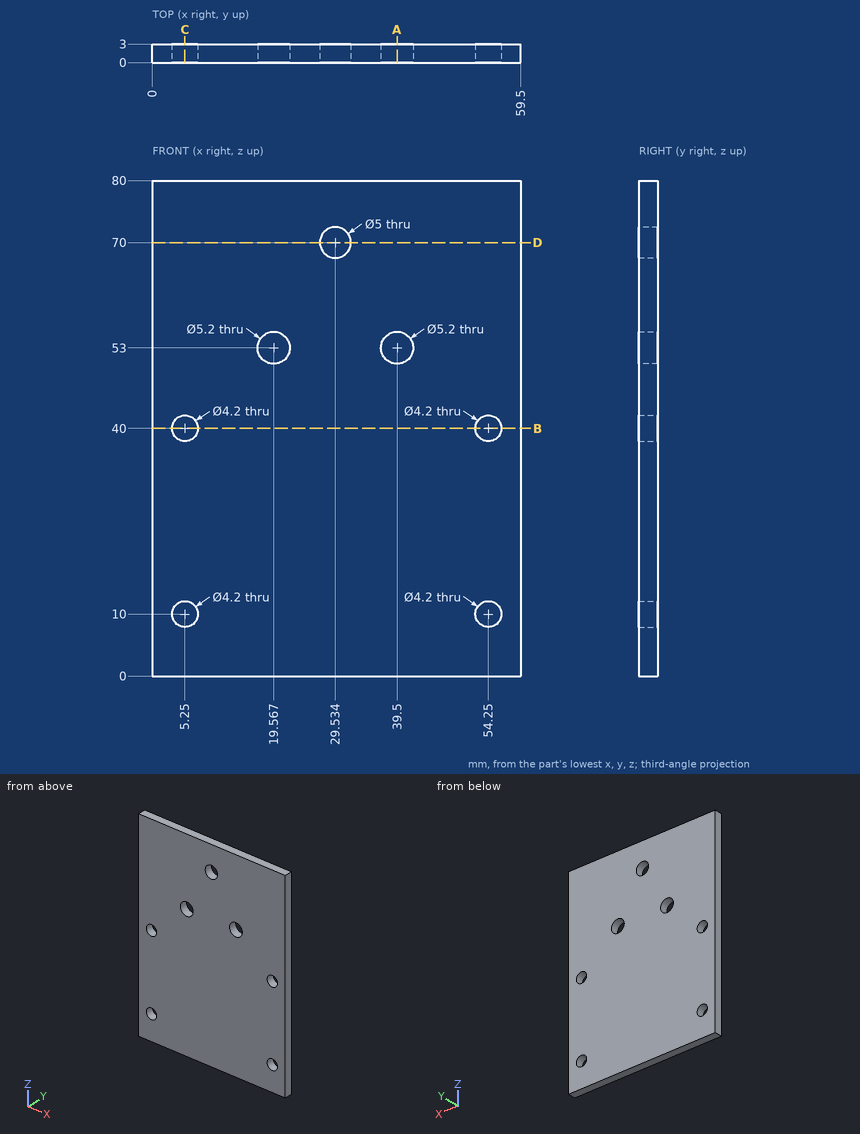
Part print with two shaded views. Sizes in mm from the minimum x, y, z corner. Coordinates: 2 decimals unless noted, no trailing zeros. Loops run counter-clockwise (first coordinate to the right, second up) from the corner with the lowest first, then second, coordinate; pieces in that order, holes last. Notation, with made-up numbers: (79.5, -11) - (124.5, -11) arc R22 ccw to (124.5, 16) - close; hole circle Ø4 at (76.25, 84). An arc over 180 degrees is marked (long way). Write each question's results on one line, items separated by ' | '. Start each with the question number.
Q1. Slice it at D-D on z = 70. Give the cut face in (x, y).
Q2. Slice it at C-C on x = 5.25. Give the cut face in (y, z).
Q3. Probe line 1 along X through (y, z) = (1, 10); line 2 along X through (y, z) = (2.35, 53); line 3 along Z through (x, y) = (54, 2.1) (1 decimal). List the from-to ranges inside material, lowest first.
Q4. Slice it at B-B on z = 40. Give the cut face in (x, y), and give its area (3 significant figures).
Q5. Slice it at A-A on x = 39.5. Give the cut face in (y, z).
Answer:
1) outline: (0, 0) - (27.03, 0) - (27.03, 3) - (0, 3) - close; (32.03, 0) - (59.5, 0) - (59.5, 3) - (32.03, 3) - close
2) outline: (0, 0) - (3, 0) - (3, 7.9) - (0, 7.9) - close; (0, 12.1) - (3, 12.1) - (3, 37.9) - (0, 37.9) - close; (0, 42.1) - (3, 42.1) - (3, 80) - (0, 80) - close
3) line 1: x = 0 to 3.15, 7.35 to 52.15, 56.35 to 59.5 | line 2: x = 0 to 16.97, 22.17 to 36.9, 42.1 to 59.5 | line 3: z = 0 to 7.9, 12.1 to 37.9, 42.1 to 80
4) outline: (0, 0) - (3.15, 0) - (3.15, 3) - (0, 3) - close; (7.35, 0) - (52.15, 0) - (52.15, 3) - (7.35, 3) - close; (56.35, 0) - (59.5, 0) - (59.5, 3) - (56.35, 3) - close | area: 153 mm2
5) outline: (0, 0) - (3, 0) - (3, 50.4) - (0, 50.4) - close; (0, 55.6) - (3, 55.6) - (3, 80) - (0, 80) - close
